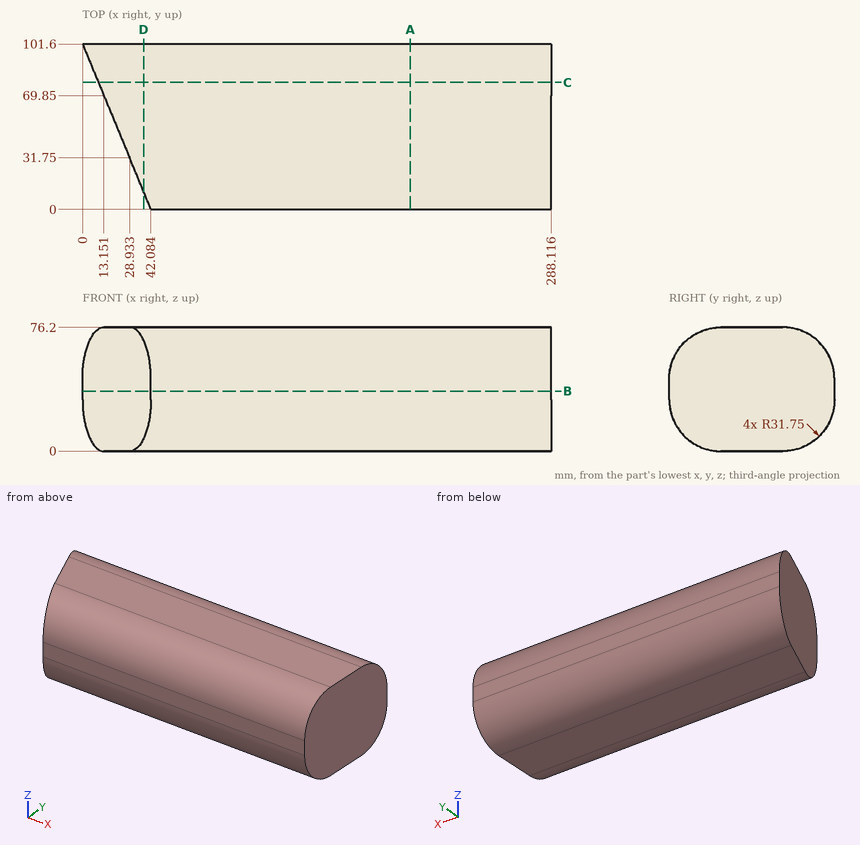
Source: three-view drawing plus pictorial views. Frame: mm from the lowest corner of the part. Give positions to 0.01 mm unless a question says otherwise; leave off trailing zeros. Write each loop counter-clockwise with the first axis right and the second up, starting at its lowest first coordinate (ties: lowest second). Pieces come first, ordered by that corner, then holes. Notation, with made-up numbers: (13, 25) - (42, 25) arc R18 cw to (42, 52) - close; hole circle Ø6 at (-21, 72). An arc over 180 degrees is marked (long way). Write item = value, one per line. Start each with the question number.
1. Section query D-D, the plane x = 37.5. Output: boundary loops of the cut face in (y, z), then the cut area to 3 significant figures.
2. First-contact query: pin 1 Ø8 at (x, z) = (60, 60) entering from +Y (1 decimal); pin 2 Ø4 at (y, z) = (33, 34.5) entering from -X; pin 3 Ø5 at (x, z) = (141.5, 29) entering from -Y. Flat tips, straight axial feed; report the tip coordinate or a pass-through.
3. Ray query, L1, parallel to Z at x = 224, y = 70.5; L2, parallel to Y at x = 169, z = 30; L3, parallel to Z at x = 234.5, y = 81. Return the intervals inside material, ascending.
4. Section query A-A, the plane x = 201.5. Output: boundary loops of the cut face in (y, z), then the cut area to 3 significant figures.
5. Section query B-B, the plane z = 37. Output: boundary loops of the cut face in (x, y), then the cut area to 3 significant figures.
6. Section query C-C, the plane y = 78. Output: boundary loops of the cut face in (x, z) (1 decimal), then the cut area to 3 significant figures.
Check sheet entries:
q1.outline = (11.07, 7.66) arc R31.75 ccw to (31.75, 0) - (69.85, 0) arc R31.75 ccw to (101.6, 31.75) - (101.6, 44.45) arc R31.75 ccw to (69.85, 76.2) - (31.75, 76.2) arc R31.75 ccw to (11.07, 68.54) - close
q1.area = 6,370 mm2
q2.pin_1 = 99.4
q2.pin_2 = 27.59
q2.pin_3 = 0
q3.L1 = 0.01 to 76.19
q3.L2 = 0.05 to 101.55
q3.L3 = 2.02 to 74.18
q4.outline = (0, 31.75) arc R31.75 ccw to (31.75, 0) - (69.85, 0) arc R31.75 ccw to (101.6, 31.75) - (101.6, 44.45) arc R31.75 ccw to (69.85, 76.2) - (31.75, 76.2) arc R31.75 ccw to (0, 44.45) - close
q4.area = 6,880 mm2
q5.outline = (0, 101.6) - (42.08, 0) - (288.12, 0) - (288.12, 101.6) - close
q5.area = 27,100 mm2
q6.outline = (9.8, 1.1) - (288.1, 1.1) - (288.1, 75.1) - (9.8, 75.1) - close
q6.area = 20,600 mm2
